Geometry check sheet. Reference: the model listing, model coordinates, mm. Face numbers are marked on the shaded views. A direction names the side the tool comes from. Give positions to 0.01 mm unless a question says otherwise; leave off trailing zeros. Loops run counter-clockwise (first coordinate to the right, second up) from the corner with the lowest first, then second, coordinate; pieces in that order, holes last. Notation, with made-up numbers: (-30, -7) -> (-9, -7) arc R11 cw to (-9, 6) -> close; hole circle Ø1 at (-8, 35). An arc over 180 degrees is marked (long way). Answer in a Markdown table with one row per item. Add a question column.
```python
from build123d import *

# Parameters (mm, degrees)
F0_R     = 11.5
F0_R_2   = 5.5
F0_R_3   = 4.05
F1_DEPTH = 1.8
F2_DEPTH = 4
F3_DEPTH = 0.7
F4_R     = 1


with BuildPart() as f1:
    # F0 (on Top) → F1 (new body)
    with BuildSketch(Plane.XY):
        Circle(F0_R)
        Circle(F0_R_2, mode=Mode.SUBTRACT)
        Circle(F0_R_2)
        Circle(F0_R_3, mode=Mode.SUBTRACT)
        Circle(F0_R_3)
    extrude(amount=-F1_DEPTH)

    # F0 (on Top) → F2 (join)
    with BuildSketch(Plane.XY):
        Circle(F0_R_3)
    extrude(amount=F2_DEPTH)

    # F0 (on Top) → F3 (join)
    with BuildSketch(Plane.XY):
        Circle(F0_R_2)
        Circle(F0_R_3, mode=Mode.SUBTRACT)
    extrude(amount=F3_DEPTH)

    # F4
    f4_edges = [f1.edges().sort_by_distance(p)[0] for p in [
        (-11.5, 0, -1.8),
    ]]
    fillet(f4_edges, radius=F4_R)


solid = f1.part
```
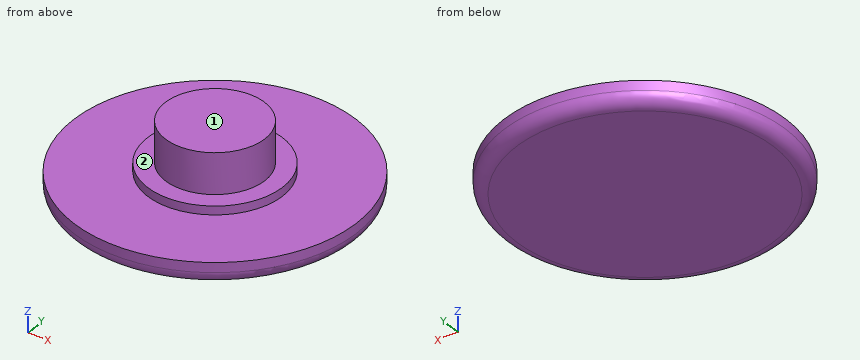
1. Gauge pin test, flat ends, axial feed: pin 1 Ø1 at (x, z) = (1, -0.5) entering from +Y; pin 2 Ø4 at (x, y) = (6, -5.5) entering from +Z. Record the tip position at first contact, or that the pin passes through.
2. Access from +Z, -Z, +X, -X, +Y, -Y to the whole of each face (thin tool, end or side, straight path). Record for the marked faces 1 and 2.
3. Material ranges on L1, parallel to Z at x = -1, y = -9.75; L2, parallel to Z at x = -2.5, y = -3.5; L3, parallel to X at y = -7, z = -0.35, recorded low to high. Write a range as from..to.
4. Sectioned sample at D-D (z = 0.35). Enter the section's corners in (x, y), plus the area to 3 significant figures.
5. Sectioned sample at C-C (z = 3.15). Enter the section's corners in (x, y).
6. Sectioned sample at A-A (x = 0). Enter the section's corners in (y, z), plus the area to 3 significant figures.
Response:
| question | item | result |
|---|---|---|
| 1 | pin 1 | stops at y = 11.49 |
| 1 | pin 2 | stops at z = 0 |
| 2 | face 1 | +Z, +X, -X, +Y, -Y |
| 2 | face 2 | +Z |
| 3 | L1 | z = -1.8..0 |
| 3 | L2 | z = -1.8..0.7 |
| 3 | L3 | x = -9.12..9.12 |
| 4 | outline | circle Ø11 at (0, 0) |
| 4 | area | 95.0 mm2 |
| 5 | outline | circle Ø8.1 at (0, 0) |
| 6 | outline | (-11.5, -0.8) arc R1 ccw to (-10.5, -1.8) -> (10.5, -1.8) arc R1 ccw to (11.5, -0.8) -> (11.5, 0) -> (5.5, 0) -> (5.5, 0.7) -> (4.05, 0.7) -> (4.05, 4) -> (-4.05, 4) -> (-4.05, 0.7) -> (-5.5, 0.7) -> (-5.5, 0) -> (-11.5, 0) -> close |
| 6 | area | 75.4 mm2 |
